Here's how the part is built. I have some questions about the finished solid (model axes, mm). A direction names the side the tool comes from. Give positions to 0.01 mm unless a question says otherwise; leave off trailing zeros. Loops run counter-clockwise (first coordinate to the right, second up) from the corner with the lowest first, then second, coordinate; pieces in that order, holes last. Notation, with made-up numbers: (10.25, 76.25) - (36.25, 76.25) arc R11 cw to (36.25, 87.25) - close; hole circle Ø7 at (3, 20.25). An arc over 180 degrees is marked (long way). Return JSON: item names as keys, results as strings. Group by question number.
(1) I need wall thicknesses on probe 1 along X at (y, z) = (-27.5, 18.5); probe 2 along X at (y, z) = (-24, 21.5); probe 3 along Z at (x, y) = (-22.25, -26.5). Which ranges of each line are inside material? Lowest first, please. Write a range as [from, to].
(2) If we section it at A-A (y = -4.5): Please give me the cut outline in (x, z).
(3) If we section it at D-D (y = -15.5): Please give me the cut outline in (x, z) (3 decimals).
(4) On a 3-axis mill with a long thin cutter (end or side, diameter ignored), from which of +Z, -Z, +X, -X, +Y, -Y can I reach the whole of each face in a straight line? I mean faces 4 (the cylindrical face through (-22.523, -22.605, 22.003)), 5 (the cylindrical face through (-30.92, 0.29, 17.37)), 6 (the cylindrical face through (-25.2, -14.7, 24.8)), 7 (the flat face through (-36.51, -15, 21)). Say none if no direction works.
(5) For P1, Ø1.9, axis at x = -40.51, y = 4, coming from the +Z side; P2, Ø1.8, axis at x = -33.5, z = 20.5, coming from the -Y side; P3, Ø1.4, axis at x = -40.5, z = 21.5, coming from the -Y side, each with a flat end and sliding along its axis, tell me the tip position at first contact or that it passes through.
(6) If we section it at B-B (z = 23.25): Please give me the cut outline in (x, y).
(7) If we section it at C-C (x = -41.25): Please give me the cut outline in (y, z), then the cut area to 3 significant figures.
(8) If we mould it in two halves opening along X, with no side actions, what happens to faces 1 (the cylindrical face through (-44.22, -11.76, 17.37)), 2 (the cylindrical face through (-38.984, 4.481, 21.13)), 3 (the flat face through (-31, 8, 21))? For each: released by +X, released by -X, zero draft, split by the parting line, or undercut.
```python
from build123d import *

# Parameters (mm, degrees)
F0_W     = 8
F0_H     = 8
F1_DEPTH = 30
F3_DEPTH = 8
F4_R     = 1.6
F5_DEPTH = 8
F7_R     = 1.375
F8_DEPTH = 15
F9_R     = 1


with BuildPart() as f1:
    # F0 (on Front) → F1 (new body)
    with BuildSketch(Plane.XZ):
        with Locations((-40.509796, 21.073834)):
            Rectangle(F0_W, F0_H)
        with Locations((-21.509796, 21.073834)):
            Rectangle(F0_W, F0_H)
    extrude(amount=F1_DEPTH)


with BuildPart() as f3:
    # F2 (on Front) → F3 (new body)
    with BuildSketch(Plane.XZ):
        Polygon((-17.509796, 25.073834), (-25.509796, 25.073834), (-36.509796, 25.073834), (-44.509796, 25.073834), (-44.509796, 17.073834), (-36.509796, 17.073834), (-25.509796, 17.073834), (-17.509796, 17.073834), align=None)
    extrude(amount=-F3_DEPTH)

    # F4 (on face) → F5 (cut, through all)
    with BuildSketch(Plane.XY.offset(25.073834)):
        with Locations((-40.509796, 4)):
            Circle(F4_R)
    extrude(amount=-F5_DEPTH, mode=Mode.SUBTRACT)


with BuildPart() as f1_1:
    add(f1.part)

    # F6: union F3
    add(f3.part)

    # F7 (on face) → F8 (cut)
    with BuildSketch(Plane.XZ.offset(30)):
        with Locations((-40.509796, 21.073834)):
            Circle(F7_R)
        with Locations((-21.509796, 21.073834)):
            Circle(F7_R)
    extrude(amount=-F8_DEPTH, mode=Mode.SUBTRACT)

    # F9
    f9_edges = [f1_1.edges().sort_by_distance(p)[0] for p in [
        (-44.509796, -11, 25.073834),
        (-36.509796, -15, 25.073834),
        (-31.009796, 0, 25.073834),
        (-31.009796, 8, 25.073834),
        (-44.509796, 8, 21.073834),
        (-31.009796, 8, 17.073834),
        (-17.509796, 8, 21.073834),
        (-25.509796, -15, 25.073834),
        (-17.509796, -11, 25.073834),
        (-17.509796, -11, 17.073834),
        (-25.509796, -15, 17.073834),
        (-31.009796, 0, 17.073834),
        (-36.509796, -15, 17.073834),
        (-44.509796, -11, 17.073834),
    ]]
    fillet(f9_edges, radius=F9_R)


solid = f1_1.part
```
Values:
{
 "1": {"probe 1": "[-44.51, -36.51], [-25.51, -17.51]", "probe 2": "[-44.51, -41.82], [-39.2, -36.51], [-25.51, -22.82], [-20.2, -17.51]", "probe 3": "[17.07, 19.92], [22.23, 25.07]"},
 "2": {"outline": "(-44.51, 18.07) arc R1 ccw to (-43.51, 17.07) - (-37.51, 17.07) arc R1 ccw to (-36.51, 18.07) - (-36.51, 24.07) arc R1 ccw to (-37.51, 25.07) - (-43.51, 25.07) arc R1 ccw to (-44.51, 24.07) - close; (-25.51, 18.07) arc R1 ccw to (-24.51, 17.07) - (-18.51, 17.07) arc R1 ccw to (-17.51, 18.07) - (-17.51, 24.07) arc R1 ccw to (-18.51, 25.07) - (-24.51, 25.07) arc R1 ccw to (-25.51, 24.07) - close"},
 "3": {"outline": "(-44.51, 18.074) arc R1 ccw to (-43.51, 17.074) - (-37.51, 17.074) arc R1 ccw to (-36.51, 18.074) - (-36.51, 24.074) arc R1 ccw to (-37.51, 25.074) - (-43.51, 25.074) arc R1 ccw to (-44.51, 24.074) - close; (-25.51, 18.074) arc R1 ccw to (-24.51, 17.074) - (-18.51, 17.074) arc R1 ccw to (-17.51, 18.074) - (-17.51, 24.074) arc R1 ccw to (-18.51, 25.074) - (-24.51, 25.074) arc R1 ccw to (-25.51, 24.074) - close; hole circle Ø2.75 at (-40.51, 21.074); hole circle Ø2.75 at (-21.51, 21.074)"},
 "4": {"face 4": "-Y", "face 5": "-Z, -Y", "face 6": "+Z, -Y", "face 7": "+Z, -Z, -Y"},
 "5": {"P1": "through", "P2": "y = 0", "P3": "y = -15"},
 "6": {"outline": "(-44.51, -30) - (-36.51, -30) - (-36.51, 0) - (-25.51, 0) - (-25.51, -30) - (-17.51, -30) - (-17.51, 7) arc R1 ccw to (-18.51, 8) - (-43.51, 8) arc R1 ccw to (-44.51, 7) - close; hole circle Ø3.2 at (-40.51, 4)"},
 "7": {"outline": "(-30, 17.07) - (2.58, 17.07) - (2.58, 25.07) - (-30, 25.07) - (-30, 22.23) - (-15, 22.23) - (-15, 19.92) - (-30, 19.92) - close; (5.42, 17.07) - (7, 17.07) arc R1 ccw to (8, 18.07) - (8, 24.07) arc R1 ccw to (7, 25.07) - (5.42, 25.07) - close", "area": "246 mm2"},
 "8": {"face 1": "released by -X", "face 2": "undercut", "face 3": "zero draft"}
}
